from build123d import *

# Parameters (mm, degrees)
PAD041_DEPTH    = 15
POCKET053_DEPTH = 13
SKETCH111_R     = 1.65
SKETCH111_R_2   = 1.7
SKETCH111_R_3   = 20
POCKET054_DEPTH = 15
POCKET055_DEPTH = 5
PAD042_DEPTH    = 55
POCKET056_DEPTH = 208.356468


with BuildPart() as part:
    # Sketch109 → Pad041 (new body)
    with BuildSketch(Plane.YZ):
        with BuildLine():
            Line((27.5, -9.253658), (27.5, -51.25))
            Line((27.5, -51.25), (-27.5, -51.25))
            Line((-27.5, -51.25), (-27.5, -9.253658))
            ThreePointArc((-20.340323, 1.39583), (-25.543681, -2.837417), (-27.5, -9.253658))
            ThreePointArc((-20.340323, 1.39583), (-18.530459, 2.868264), (-17.85, 5.1))
            ThreePointArc((-12.15, 5.1), (-15, 7.95), (-17.85, 5.1))
            ThreePointArc((-12.15, 5.1), (-11.315254, 3.084746), (-9.3, 2.25))
            Line((-9.3, 2.25), (9.3, 2.25))
            ThreePointArc((9.3, 2.25), (11.315254, 3.084746), (12.15, 5.1))
            ThreePointArc((17.85, 5.1), (15, 7.95), (12.15, 5.1))
            ThreePointArc((17.85, 5.1), (18.530459, 2.868264), (20.340323, 1.39583))
            ThreePointArc((27.5, -9.253658), (25.543681, -2.837417), (20.340323, 1.39583))
        make_face()
    extrude(amount=-PAD041_DEPTH)

    # Sketch110 (on Face14 of Pad041) → Pocket053 (cut)
    with BuildSketch(Plane(origin=(-15, 0, 0), x_dir=(0, -1, 0), z_dir=(-1, 0, 0))):
        with BuildLine():
            Line((-26, -9.253658), (-26, -51.25))
            Line((-26, -51.25), (26, -51.25))
            Line((26, -51.25), (26, -9.253658))
            ThreePointArc((26, -9.253658), (23.071068, -2.18259), (16, 0.746342))
            Line((-16, 0.746342), (16, 0.746342))
            ThreePointArc((-16, 0.746342), (-23.071068, -2.18259), (-26, -9.253658))
        make_face()
    extrude(amount=-POCKET053_DEPTH, mode=Mode.SUBTRACT)

    # Sketch111 (on Face4 of Pocket053) → Pocket054 (cut)
    with BuildSketch(Plane.YZ):
        with Locations((-15, 5.1)):
            Circle(SKETCH111_R)
        with Locations((15, 5.1)):
            Circle(SKETCH111_R)
        with Locations((22.4, -44.05)):
            Circle(SKETCH111_R_2)
        with Locations((-20.9, -5.25)):
            Circle(SKETCH111_R_2)
        with Locations((2, -26.25)):
            Circle(SKETCH111_R_3)
    extrude(amount=-POCKET054_DEPTH, mode=Mode.SUBTRACT)

    # Sketch112 (on Face11 of Pocket054) → Pocket055 (cut)
    with BuildSketch(Plane(origin=(0, -27.5, 0), x_dir=(0, 0, 1), z_dir=(0, -1, 0))):
        Polygon((-51.25, 15), (-28.815971, 15), (-38.35, 7), (-51.25, 7), align=None)
    extrude(amount=-POCKET055_DEPTH, mode=Mode.SUBTRACT)

    # Sketch114 (on Face7 of Pocket055) → Pad042 (join)
    with BuildSketch(Plane.XZ.offset(-27.5)):
        with BuildLine():
            ThreePointArc((-5.864892, -58.75), (-1.6403, -56.01044), (0, -51.25))
            Line((0, -51.25), (-17, -51.25))
            Line((-17, -51.25), (-36.926579, -64))
            Line((-36.926579, -64), (-27, -64))
            Line((-27, -64), (-5.864892, -58.75))
        make_face()
    extrude(amount=PAD042_DEPTH)

    # Sketch115 (on Face20 of Pad042) → Pocket056 (cut, through all)
    with BuildSketch(Plane(origin=(0, 0, -51.25), x_dir=(0, -1, 0), z_dir=(0, 0, 1))):
        with BuildLine():
            Line((-27.5, -17), (-27.5, -43))
            Line((-27.5, -43), (0, -43))
            Line((0, -43), (0, -17))
            Line((0, -17), (-15.050161, -17))
            ThreePointArc((-15.050161, -17), (-14.226455, -19.908295), (-12, -21.952695))
            Line((-12, -21.952695), (-15.2, -32.476953))
            ThreePointArc((-27.5, -17), (-24.05052, -26.884661), (-15.2, -32.476953))
        make_face()
    pocket056 = extrude(amount=-POCKET056_DEPTH, mode=Mode.SUBTRACT)

    # Mirrored001: Pocket056 across Sketch115 V_Axis
    add(pocket056.mirror(Plane(origin=(0, 0, -51.25), x_dir=(0, 0, 1), z_dir=(0, -1, 0))), mode=Mode.SUBTRACT)


with BuildPart() as part_1:
    # Body015 placement: moved
    add(part.part.moved(Location((32, 0, 0))))


solid = part_1.part
The model under review builds one solid part; all positions refer to its coordinate system, in mm. A direction names the side the tool comes from. Give positions to 0.01 mm unless a question says otherwise; leave off trailing zeros. Order: outer loops, then holes, each group sorted by start corner. A loop starts at its lowest first (then second) coordinate and runs counter-clockwise, first axis right, second up. Notation, with made-up numbers: M 76.5,50.25 L 133.5,50.25 A28 ccw 133.5,68.25 Z; hole C -8.5,39 d10. An arc over 180 degrees is marked long. Use one line per item in the form item = value. Start each with the question number.
Item 1: We need section B-B on y = 2. Give the boundary of the cut face in (x, z).
Item 2: We need section A-A on z = -26.25. Give the boundary of the cut face in (x, y), plus the area to 3 significant figures.
Item 3: For faces 4 (the flat face through (25, 0, 2.25)), 5 (the flat face through (23, 0, 0.746)), 6 (the flat face through (25, -27, -45)), 7 (the cylindrical face through (12.13, -14.25, -58.2)), list the 3-axis set-ups (+Z, -Z, +X, -X, +Y, -Y) from which the entire face can be reached by the end or side of a thin tool; tool diameter is ignored.
Item 4: To check wall thickness, follow line 1 along Y through (x, z) = (24, 5); line 2 along Y through (x, z) = (31, -26); line 3 along Y through (x, z) = (26, 4). State the ranges of each line that lie inside material, in increasing order. Write a range as from..to.
Item 5: Insertion check: pin 1 Ø11.5 at (y, z) = (-5.5, -58) entering from -X; pin 2 Ø2.5 at (y, z) = (-20.9, -5.25) entering from -X; pin 3 Ø4 at (x, y) = (26, -1) entering from -Z; pin 4 Ø7.5 at (x, y) = (20.5, -2.5) entering from +Z. Each pin has a flat end and moves straight along its axis. Give the tip position at first contact, or say it passes through.
Item 6: The part is to be moulded in two halves that separate along Z. For faces 1 (the cylindrical face through (23.41, -23.15, -2.26)), 2 (the flat face through (25, -27.5, -35)), 3 (the cylindrical face through (24.6, 18.51, 2.9)), say which applies: pulls with the +Z half, pulls with the -Z half, needs draft (parallel to the pull), parting line crosses it, or undercut.
Item 7: We need section C-C on z = -49.5. Give the boundary of the cut face in (x, y).
Item 8: We need section D-D on y = -4.5. Give the boundary of the cut face in (x, z), plus the area to 3 significant figures.
Completed:
q1.outline = M 15,-61.52 L 26.14,-58.75 A7.73 ccw 32,-51.25 L 32,-46.25 L 30,-46.25 L 30,-51.25 L 15,-51.25 Z; M 17,0.75 L 30,0.75 L 30,-6.25 L 32,-6.25 L 32,2.25 L 17,2.25 Z
q2.outline = M 17,-27.5 L 32,-27.5 L 32,-18 L 30,-18 L 30,-26 L 17,-26 Z; M 17,26 L 30,26 L 30,22 L 32,22 L 32,27.5 L 17,27.5 Z
q2.area = 69.0 mm²
q3.face_4 = +Z, +X, -X
q3.face_5 = -X
q3.face_6 = -X, -Y
q3.face_7 = +Z, -Z
q4.line_1 = -17.85..-16.65, -13.35..-12.15, 12.15..13.35, 16.65..17.85
q4.line_2 = -27.5..-18, 22..27.5
q4.line_3 = -18..-16.23, -13.77..-11.93, 11.93..13.77, 16.23..18
q5.pin_1 = 15
q5.pin_2 = through
q5.pin_3 = -59.28
q5.pin_4 = 2.25
q6.face_1 = undercut
q6.face_2 = needs draft
q6.face_3 = pulls with the +Z half
q7.outline = M 17,26 L 30,26 L 30,-26 L 25,-26 L 25,-27.5 L 32,-27.5 L 32,27.5 L 17,27.5 Z
q8.outline = M 15,-61.52 L 26.14,-58.75 A7.73 ccw 32,-51.25 L 32,-45.16 L 30,-45.16 L 30,-51.25 L 15,-51.25 Z; M 17,0.75 L 30,0.75 L 30,-7.34 L 32,-7.34 L 32,2.25 L 17,2.25 Z
q8.area = 182 mm²
